from build123d import *

# Parameters (mm, degrees)
F0_W      = 160
F0_H      = 125
F1_DEPTH  = 16.5
F4_W      = 37
F4_H      = 10.5
F6_W      = 10.5
F6_H      = 20
F6_H_2    = 21
F8_W      = 35
F8_H      = 10.5
F10_W     = 10.5
F10_H     = 21
F12_W     = 10.5
F12_H     = 21
F16_R     = 8.5
F17_DEPTH = 8
F18_W     = 160
F18_H     = 5
F19_DEPTH = 160
F20_W     = 1.2669073437
F20_H     = 18.4661853126
F20_W_2   = 18.4661853126
F20_H_2   = 1.2669073437
F21_DEPTH = 5


with BuildPart() as f1:
    # F0 (on Top) → F1 (new body)
    with BuildSketch(Plane.XY):
        with Locations((80, 62.5)):
            Rectangle(F0_W, F0_H)
    extrude(amount=-F1_DEPTH)

    # F2 (on face) → F3 (revolve, cut)
    with BuildSketch(Plane.XY):
        Polygon((20, 75), (20, 60), (27, 60), (27, 75), (35.5, 75), (35.5, 85), (32, 85), (32, 99), (24.5, 99), (24.5, 113), (20, 113), (20, 99), (20, 85), align=None)
    revolve(axis=Axis((20, 92, 0), (0, 1, 0)), mode=Mode.SUBTRACT)

    # F4 (on face) → F5 (revolve, cut)
    with BuildSketch(Plane.XY):
        with Locations((58.5, 69.75)):
            Rectangle(F4_W, F4_H)
    revolve(axis=Axis((58.5, 75, 0), (1, 0, 0)), mode=Mode.SUBTRACT)

    # F6 (on face) → F7 (revolve, cut)
    with BuildSketch(Plane.XY):
        with Locations((71.75, 95.5)):
            Rectangle(F6_W, F6_H)
        with Locations((71.75, 75)):
            Rectangle(F6_W, F6_H_2)
    revolve(axis=Axis((66.5, 85, 0), (0, 1, 0)), mode=Mode.SUBTRACT)

    # F8 (on face) → F9 (revolve, cut)
    with BuildSketch(Plane.XY):
        with Locations((99.5, 72.75)):
            Rectangle(F8_W, F8_H)
        with Locations((139.5, 72.75)):
            Rectangle(F8_W, F8_H)
    revolve(axis=Axis((99.5, 78, 0), (1, 0, 0)), mode=Mode.SUBTRACT)

    # F10 (on face) → F11 (revolve, cut)
    with BuildSketch(Plane.XY):
        Polygon((106.5, 88.5), (117, 88.5), (117, 94.5), (113, 98.5), (106.5, 98.5), align=None)
        with Locations((111.75, 78)):
            Rectangle(F10_W, F10_H)
    revolve(axis=Axis((106.5, 83, 0), (0, 1, 0)), mode=Mode.SUBTRACT)

    # F12 (on face) → F13 (revolve, cut)
    with BuildSketch(Plane.XY):
        Polygon((146.5, 88.5), (157, 88.5), (157, 94.5), (153, 98.5), (146.5, 98.5), align=None)
        with Locations((151.75, 78)):
            Rectangle(F12_W, F12_H)
    revolve(axis=Axis((146.5, 83, 0), (0, 1, 0)), mode=Mode.SUBTRACT)

    # F14 (on face) → F15 (revolve, cut)
    with BuildSketch(Plane.XY):
        Polygon((20, 13.5), (20, 5), (27, 5), (27, 13.5), (32.5, 13.5), (32.5, 28), (29, 28), (29, 41), (20, 41), (20, 28), align=None)
    revolve(axis=Axis((20, 20.75, 0), (0, 1, 0)), mode=Mode.SUBTRACT)

    # F16 (on face) → F17 (cut)
    with BuildSketch(Plane.XY):
        with Locations((56, 21)):
            Circle(F16_R)
    extrude(amount=-F17_DEPTH, mode=Mode.SUBTRACT)

    # F18 (on face) → F19 (cut)
    with BuildSketch(Plane.XZ):
        with Locations((80, -2.5)):
            Rectangle(F18_W, F18_H)
    extrude(amount=-F19_DEPTH, mode=Mode.SUBTRACT)

    # F20 (on face) → F21 (join)
    with BuildSketch(Plane.XY.offset(-5)):
        with Locations((76.3665463282, 75)):
            Rectangle(F20_W, F20_H)
        with Locations((66.5, 65.1334536718)):
            Rectangle(F20_W_2, F20_H_2)
        with Locations((116.3665463282, 78)):
            Rectangle(F20_W, F20_H)
        with Locations((106.5, 68.1334536718)):
            Rectangle(F20_W_2, F20_H_2)
        with Locations((156.3665463282, 78)):
            Rectangle(F20_W, F20_H)
        with Locations((146.5, 68.1334536718)):
            Rectangle(F20_W_2, F20_H_2)
    extrude(amount=-F21_DEPTH)


solid = f1.part
Input: part model. Units: mm. Frame: model coordinates. A direction names the side the tool comes from. Round coordinates to 2 decimals unless told otherwise and drop trailing zeros. Write each loop counter-clockwise with the first axis right and the second up, starting at its lowest first coordinate (ties: lowest second). Pieces come first, ordered by that corner, then holes.
1) Cut plane A-A (x = 90). Return the cut outline in (y, z).
2) Cut plane B-B (y = 21). Return the cut outline in (x, z), then the cut area to 3 significant figures.
3) Reachability of faces 5 (the cylindrical face through (50.5, 74.8, -10.5)), 6 (the flat face through (79, 63, -16.5)) from +Z, -Z, +X, -X, +Y, -Y: full face, straight path, thin tool, end or side. Return the list, or none.
4) Ray query, L1, parallel to Y at x = 56, z = -7.3; L2, parallel to X at y = 14, z = -6.75; L3, parallel to Y at x = 56, z = -5.7. Return the intervals inside material, ascending.
5) Cut plane C-C (x = 51). Return the cut outline in (y, z).
6) Draft query along Y for faces 1 (the flat face through (79, 125, -11)), 2 (the flat face through (56, 21, -8)), 3 (the flat face through (160, 62, -11)), 4 (the cylindrical face through (49.255, 15.828, -6.479)). Return one class per face: pulls with the +Y half, pulls with the -Y half, needs draft (parallel to the pull), parting line crosses it, or undercut.
Geometry says:
1. outline: (0, -16.5) - (125, -16.5) - (125, -5) - (87.23, -5) arc R10.5 cw to (68.77, -5) - (0, -5) - close
2. outline: (0, -16.5) - (160, -16.5) - (160, -5) - (64.5, -5) - (64.5, -8) - (47.5, -8) - (47.5, -5) - (31.46, -5) arc R12.5 cw to (8.54, -5) - (0, -5) - close
2. area: 1,670 mm2
3. face 5: +Z
3. face 6: -Z, +X, -X, +Y, -Y
4. L1: y = 0 to 12.5, 29.5 to 67.45, 82.55 to 125
4. L2: x = 0 to 9.48, 30.52 to 51.18, 60.82 to 160
4. L3: y = 0 to 12.5, 29.5 to 66.18, 83.82 to 125
5. outline: (0, -16.5) - (125, -16.5) - (125, -5) - (84.23, -5) arc R10.5 cw to (65.77, -5) - (27.87, -5) - (27.87, -8) - (14.13, -8) - (14.13, -5) - (0, -5) - close
6. face 1: pulls with the +Y half
6. face 2: undercut
6. face 3: needs draft
6. face 4: undercut
